from build123d import *

# Parameters (mm, degrees)
BOSS_EXTRUDE1_START       = -0.6
BOSS_EXTRUDE1_DEPTH       = 3.3
BOSS_EXTRUDE1_2_OUTLINE_W = 9.5
BOSS_EXTRUDE1_2_OUTLINE_H = 2.8
BOSS_EXTRUDE1_2_DEPTH     = 0.6
BOSS_EXTRUDE1_3_OUTLINE_R = 0.25
BOSS_EXTRUDE1_3_ANGLE     = 48.590678
SKETCH2_W                 = 12
SKETCH2_H                 = 5
SKETCH2_W_2               = 0.7
SKETCH2_H_2               = 1
BOSS_EXTRUDE2_DEPTH       = 0.4
SKETCH3_W                 = 2.7
SKETCH3_H                 = 9.5
CUT_EXTRUDE1_DEPTH        = 0.6
SKETCH4_W                 = 0.45
SKETCH4_H                 = 1.7
CUT_EXTRUDE2_DEPTH        = 15.612665805
CUT_EXTRUDE3_REACH        = 50.095
SKETCH6_W                 = 0.05
SKETCH6_H                 = 1.7
SKETCH7_W                 = 0.45
SKETCH7_H                 = 1.7
CUT_EXTRUDE4_DEPTH        = 15.612665805
CUT_EXTRUDE5_REACH        = 50.095
SKETCH9_W                 = 0.05
SKETCH9_H                 = 1.7
CUT_EXTRUDE6_REACH        = 50.095
SKETCH11_W                = 0.75
SKETCH11_H                = 0.1
SKETCH12_W                = 0.2
SKETCH12_H                = 1.5
BOSS_EXTRUDE3_DEPTH       = 0.4
CUT_EXTRUDE7_REACH        = 50.095
SKETCH14_W                = 0.75
SKETCH14_H                = 0.1
CUT_EXTRUDE8_REACH        = 50.095
SKETCH16_W                = 0.75
SKETCH16_H                = 0.1
SKETCH17_W                = 0.2
SKETCH17_H                = 1.5
BOSS_EXTRUDE4_DEPTH       = 0.4
CUT_EXTRUDE9_REACH        = 50.095
SKETCH19_W                = 0.75
SKETCH19_H                = 0.1
BOSS_EXTRUDE5_DEPTH       = 9.5
SKETCH21_W                = 0.8
SKETCH21_H                = 0.6
CUT_EXTRUDE10_DEPTH       = 1.8
SKETCH22_W                = 0.8
SKETCH22_H                = 0.6
CUT_EXTRUDE11_DEPTH       = 1.8
SKETCH23_R                = 0.25
BOSS_EXTRUDE6_DEPTH       = 1.35
SKETCH24_R                = 0.25
BOSS_EXTRUDE7_DEPTH       = 1.35
SKETCH25_R                = 0.25
BOSS_EXTRUDE8_DEPTH       = 1.35
SKETCH26_R                = 0.25
BOSS_EXTRUDE9_DEPTH       = 1.35
SKETCH27_R                = 0.25
BOSS_EXTRUDE10_DEPTH      = 1.35
BOSS_EXTRUDE11_DEPTH      = 0.5
BOSS_EXTRUDE12_DEPTH      = 0.5
SKETCH30_R                = 0.25
BOSS_EXTRUDE13_DEPTH      = 1.35
SKETCH31_W                = 0.25
SKETCH31_H                = 2.4
SKETCH32_W                = 0.25
SKETCH32_H                = 2.4
SKETCH33_W                = 0.25
SKETCH33_H                = 2.4
SKETCH34_W                = 0.25
SKETCH34_H                = 2.4
SKETCH35_W                = 0.25
SKETCH35_H                = 2.4
SKETCH36_W                = 0.25
SKETCH36_H                = 2.4


with BuildPart() as part:
    # Boss-Extrude1: read off the stored shape, not the designer's step
    # Boss-Extrude1 outline → Boss-Extrude1 (new body)
    with BuildSketch(Plane(origin=(41.85, 0, 0), x_dir=(0, 0, -1), z_dir=(1, 0, 0)).offset(BOSS_EXTRUDE1_START)):
        Polygon((-4.75, 12.8), (-6, 12.8), (-6, 7.8), (6, 7.8), (6, 12.8), (4.75, 12.8), (4.75, 10), (-4.75, 10), align=None)
    extrude(amount=BOSS_EXTRUDE1_DEPTH)

    # Boss-Extrude1 2 outline → Boss-Extrude1 2 (add)
    with BuildSketch(Plane(origin=(41.85, 0, 0), x_dir=(0, 0, -1), z_dir=(1, 0, 0)).offset(BOSS_EXTRUDE1_START)):
        with Locations((0, 11.4)):
            Rectangle(BOSS_EXTRUDE1_2_OUTLINE_W, BOSS_EXTRUDE1_2_OUTLINE_H)
    extrude(amount=BOSS_EXTRUDE1_2_DEPTH)

    # Boss-Extrude1 3 outline → Boss-Extrude1 3 (revolve)
    with BuildSketch(Plane(origin=(41.95, 7.65, 0), x_dir=(-0.6614338946121362, 0.7500034686974597, 0), z_dir=(0.7500034686974597, 0.6614338946121362, 0))):
        with Locations((0.45, 2.25)):
            Circle(BOSS_EXTRUDE1_3_OUTLINE_R)
        with Locations((0.45, -2.25)):
            Circle(BOSS_EXTRUDE1_3_OUTLINE_R)
        with Locations((0.45, -0.75)):
            Circle(BOSS_EXTRUDE1_3_OUTLINE_R)
        with Locations((0.45, 0.75)):
            Circle(BOSS_EXTRUDE1_3_OUTLINE_R)
        with Locations((0.45, 3.75)):
            Circle(BOSS_EXTRUDE1_3_OUTLINE_R)
        with Locations((0.45, -3.75)):
            Circle(BOSS_EXTRUDE1_3_OUTLINE_R)
    revolve(axis=Axis((41.95, 7.65, 0), (0, 0, 1)), revolution_arc=BOSS_EXTRUDE1_3_ANGLE)

    # Sketch2 → Boss-Extrude2 (add)
    with BuildSketch(Plane(origin=(44.55, 0, 0), x_dir=(0, 0, -1), z_dir=(1, 0, 0))):
        with Locations((0, 10.3)):
            Rectangle(SKETCH2_W, SKETCH2_H)
        with Locations((4.4, 10.5)):
            Rectangle(SKETCH2_W_2, SKETCH2_H_2, mode=Mode.SUBTRACT)
        with Locations((-4.4, 10.5)):
            Rectangle(SKETCH2_W_2, SKETCH2_H_2, mode=Mode.SUBTRACT)
    extrude(amount=BOSS_EXTRUDE2_DEPTH)

    # Sketch3 → Cut-Extrude1 (cut)
    with BuildSketch(Plane(origin=(0, 10, 0), x_dir=(-1, 0, 0), z_dir=(0, 1, 0))):
        with Locations((-43.2, 0)):
            Rectangle(SKETCH3_W, SKETCH3_H)
    extrude(amount=-CUT_EXTRUDE1_DEPTH, mode=Mode.SUBTRACT)

    # Sketch4 → Cut-Extrude2 (cut, through all)
    with BuildSketch(Plane(origin=(44.95, 0, 0), x_dir=(0, 0, -1), z_dir=(1, 0, 0))):
        with Locations((-5.775, 10.85)):
            Rectangle(SKETCH4_W, SKETCH4_H)
    extrude(amount=-CUT_EXTRUDE2_DEPTH, mode=Mode.SUBTRACT)

    # Sketch6 → Cut-Extrude3 (cut, up to next)
    with BuildSketch(Plane(origin=(0, 0, 5.35), x_dir=(-1, 0, 0), z_dir=(0, 0, -1)), mode=Mode.PRIVATE) as cut_extrude3_sk1:
        with Locations((-44.925, 10.85)):
            Rectangle(SKETCH6_W, SKETCH6_H)
    cut_extrude3_tool1 = extrude(cut_extrude3_sk1.sketch, amount=-CUT_EXTRUDE3_REACH, mode=Mode.PRIVATE) & part.part
    add(cut_extrude3_tool1.solids().sort_by_distance((44.925, 10.85, 5.35))[0], mode=Mode.SUBTRACT)

    # Sketch7 → Cut-Extrude4 (cut, through all)
    with BuildSketch(Plane(origin=(44.95, 0, 0), x_dir=(0, 0, -1), z_dir=(1, 0, 0))):
        with Locations((5.775, 10.85)):
            Rectangle(SKETCH7_W, SKETCH7_H)
    extrude(amount=-CUT_EXTRUDE4_DEPTH, mode=Mode.SUBTRACT)

    # Sketch9 → Cut-Extrude5 (cut, up to next)
    with BuildSketch(Plane.XY.offset(-5.35), mode=Mode.PRIVATE) as cut_extrude5_sk1:
        with Locations((44.925, 10.85)):
            Rectangle(SKETCH9_W, SKETCH9_H)
    cut_extrude5_tool1 = extrude(cut_extrude5_sk1.sketch, amount=-CUT_EXTRUDE5_REACH, mode=Mode.PRIVATE) & part.part
    add(cut_extrude5_tool1.solids().sort_by_distance((44.925, 10.85, -5.35))[0], mode=Mode.SUBTRACT)

    # Sketch11 → Cut-Extrude6 (cut, up to next)
    with BuildSketch(Plane.XY.offset(-5.35), mode=Mode.PRIVATE) as cut_extrude6_sk1:
        with Locations((41.625, 10.05)):
            Rectangle(SKETCH11_W, SKETCH11_H)
    cut_extrude6_tool1 = extrude(cut_extrude6_sk1.sketch, amount=-CUT_EXTRUDE6_REACH, mode=Mode.PRIVATE) & part.part
    add(cut_extrude6_tool1.solids().sort_by_distance((41.625, 10.05, -5.35))[0], mode=Mode.SUBTRACT)

    # Sketch12 → Boss-Extrude3 (add)
    with BuildSketch(Plane(origin=(0, 0, -5.55), x_dir=(-1, 0, 0), z_dir=(0, 0, -1))):
        with Locations((-41.35, 10.85)):
            Rectangle(SKETCH12_W, SKETCH12_H)
    extrude(amount=BOSS_EXTRUDE3_DEPTH)

    # Sketch14 → Cut-Extrude7 (cut, up to next)
    with BuildSketch(Plane.XY.offset(-5.35), mode=Mode.PRIVATE) as cut_extrude7_sk1:
        with Locations((41.625, 11.65)):
            Rectangle(SKETCH14_W, SKETCH14_H)
    cut_extrude7_tool1 = extrude(cut_extrude7_sk1.sketch, amount=-CUT_EXTRUDE7_REACH, mode=Mode.PRIVATE) & part.part
    add(cut_extrude7_tool1.solids().sort_by_distance((41.625, 11.65, -5.35))[0], mode=Mode.SUBTRACT)

    # Sketch16 → Cut-Extrude8 (cut, up to next)
    with BuildSketch(Plane(origin=(0, 0, 5.35), x_dir=(-1, 0, 0), z_dir=(0, 0, -1)), mode=Mode.PRIVATE) as cut_extrude8_sk1:
        with Locations((-41.625, 11.65)):
            Rectangle(SKETCH16_W, SKETCH16_H)
    cut_extrude8_tool1 = extrude(cut_extrude8_sk1.sketch, amount=-CUT_EXTRUDE8_REACH, mode=Mode.PRIVATE) & part.part
    add(cut_extrude8_tool1.solids().sort_by_distance((41.625, 11.65, 5.35))[0], mode=Mode.SUBTRACT)

    # Sketch17 → Boss-Extrude4 (add)
    with BuildSketch(Plane.XY.offset(5.55)):
        with Locations((41.35, 10.85)):
            Rectangle(SKETCH17_W, SKETCH17_H)
    extrude(amount=BOSS_EXTRUDE4_DEPTH)

    # Sketch19 → Cut-Extrude9 (cut, up to next)
    with BuildSketch(Plane(origin=(0, 0, 5.35), x_dir=(-1, 0, 0), z_dir=(0, 0, -1)), mode=Mode.PRIVATE) as cut_extrude9_sk1:
        with Locations((-41.625, 10.05)):
            Rectangle(SKETCH19_W, SKETCH19_H)
    cut_extrude9_tool1 = extrude(cut_extrude9_sk1.sketch, amount=-CUT_EXTRUDE9_REACH, mode=Mode.PRIVATE) & part.part
    add(cut_extrude9_tool1.solids().sort_by_distance((41.625, 10.05, 5.35))[0], mode=Mode.SUBTRACT)

    # Sketch20 → Boss-Extrude5 (add)
    with BuildSketch(Plane(origin=(0, 0, 4.75), x_dir=(-1, 0, 0), z_dir=(0, 0, -1))):
        Polygon((-42.9, 9.4), (-44.55, 9.4), (-44.55, 9.7), (-43.2, 9.7), align=None)
    extrude(amount=BOSS_EXTRUDE5_DEPTH)

    # Sketch21 → Cut-Extrude10 (cut)
    with BuildSketch(Plane(origin=(0, 12.8, 0), x_dir=(-1, 0, 0), z_dir=(0, 1, 0))):
        with Locations((-43.65, -5.05)):
            Rectangle(SKETCH21_W, SKETCH21_H)
    extrude(amount=-CUT_EXTRUDE10_DEPTH, mode=Mode.SUBTRACT)

    # Sketch22 → Cut-Extrude11 (cut)
    with BuildSketch(Plane(origin=(0, 12.8, 0), x_dir=(-1, 0, 0), z_dir=(0, 1, 0))):
        with Locations((-43.65, 5.05)):
            Rectangle(SKETCH22_W, SKETCH22_H)
    extrude(amount=-CUT_EXTRUDE11_DEPTH, mode=Mode.SUBTRACT)

    # Sketch23 → Boss-Extrude6 (add)
    with BuildSketch(Plane.XZ.offset(-7.65)):
        with Locations(Location((41.5, 2.25, 0), (0, 0, 90))):
            Circle(SKETCH23_R)
    extrude(amount=BOSS_EXTRUDE6_DEPTH)

    # Sketch24 → Boss-Extrude7 (add)
    with BuildSketch(Plane.XZ.offset(-7.65)):
        with Locations(Location((41.5, -0.75, 0), (0, 0, 90))):
            Circle(SKETCH24_R)
    extrude(amount=BOSS_EXTRUDE7_DEPTH)

    # Sketch25 → Boss-Extrude8 (add)
    with BuildSketch(Plane.XZ.offset(-7.65)):
        with Locations(Location((41.5, -3.75, 0), (0, 0, 90))):
            Circle(SKETCH25_R)
    extrude(amount=BOSS_EXTRUDE8_DEPTH)

    # Sketch26 → Boss-Extrude9 (add)
    with BuildSketch(Plane.XZ.offset(-7.65)):
        with Locations(Location((41.5, -2.25, 0), (0, 0, 90))):
            Circle(SKETCH26_R)
    extrude(amount=BOSS_EXTRUDE9_DEPTH)

    # Sketch27 → Boss-Extrude10 (add)
    with BuildSketch(Plane.XZ.offset(-7.65)):
        with Locations(Location((41.5, 0.75, 0), (0, 0, 90))):
            Circle(SKETCH27_R)
    extrude(amount=BOSS_EXTRUDE10_DEPTH)

    # Sketch28 → Boss-Extrude11 (add)
    with BuildSketch(Plane.XY.offset(6)):
        Polygon((43.35, 7.8), (41.25, 7.8), (41.25, 6.8), (42.75, 6.8), align=None)
    extrude(amount=-BOSS_EXTRUDE11_DEPTH)

    # Sketch29 → Boss-Extrude12 (add)
    with BuildSketch(Plane(origin=(0, 0, -6), x_dir=(-1, 0, 0), z_dir=(0, 0, -1))):
        Polygon((-41.25, 6.8), (-41.25, 7.8), (-43.35, 7.8), (-42.75, 6.8), align=None)
    extrude(amount=-BOSS_EXTRUDE12_DEPTH)

    # Sketch30 → Boss-Extrude13 (add)
    with BuildSketch(Plane.XZ.offset(-7.65)):
        with Locations(Location((41.5, 3.75, 0), (0, 0, 90))):
            Circle(SKETCH30_R)
    extrude(amount=BOSS_EXTRUDE13_DEPTH)

    # Sketch31 → Revolve1 (revolve)
    with BuildSketch(Plane.XY.offset(3.75)):
        with Locations((43.775, 10.9)):
            Rectangle(SKETCH31_W, SKETCH31_H)
    revolve(axis=Axis((43.65, 12.1, 3.75), (0, -1, 0)))

    # Sketch32 → Revolve2 (revolve)
    with BuildSketch(Plane.XY.offset(0.75)):
        with Locations((43.775, 10.9)):
            Rectangle(SKETCH32_W, SKETCH32_H)
    revolve(axis=Axis((43.65, 12.1, 0.75), (0, -1, 0)))

    # Sketch33 → Revolve3 (revolve)
    with BuildSketch(Plane.XY.offset(-2.25)):
        with Locations((43.775, 10.9)):
            Rectangle(SKETCH33_W, SKETCH33_H)
    revolve(axis=Axis((43.65, 12.1, -2.25), (0, -1, 0)))

    # Sketch34 → Revolve4 (revolve)
    with BuildSketch(Plane.XY.offset(-3.75)):
        with Locations((43.775, 10.9)):
            Rectangle(SKETCH34_W, SKETCH34_H)
    revolve(axis=Axis((43.65, 12.1, -3.75), (0, -1, 0)))

    # Sketch35 → Revolve5 (revolve)
    with BuildSketch(Plane.XY.offset(-0.75)):
        with Locations((43.775, 10.9)):
            Rectangle(SKETCH35_W, SKETCH35_H)
    revolve(axis=Axis((43.65, 12.1, -0.75), (0, -1, 0)))

    # Sketch36 → Revolve6 (revolve)
    with BuildSketch(Plane.XY.offset(2.25)):
        with Locations((43.775, 10.9)):
            Rectangle(SKETCH36_W, SKETCH36_H)
    revolve(axis=Axis((43.65, 12.1, 2.25), (0, -1, 0)))


solid = part.part
Source: CAD feature listing. Evaluate the final solid. Frame: model axes, mm. A direction names the side the tool comes from. Round coordinates to 2 decimals unless told otherwise and drop trailing zeros. Write each loop counter-clockwise with the first axis right and the second up, starting at its lowest first coordinate (ties: lowest second). Pieces come first, ordered by that corner, then holes. Notation, with made-up numbers: M 25.25,21.5 L 34.25,21.5 A17 ccw 34.25,54.5 Z; hole C -39,-28.5 d5. An arc over 180 degrees is marked long. One line per item, written item: value. Start each with the question number.
Item 1: Set-up query: faces 1 (the flat face through (43, 11, -5.55)), 2 (the flat face through (43, 11, 5.55)), 3 (the flat face through (42, 7, -5.5)), 4 (the flat face through (44, 9.7, 0)). Return all of +Z, -Z, +X, -X, +Y, -Y with unobstructed straight access to the full face (end or side cutting, diameter ignored); none if empty.
Item 2: Mould query, pull axis Z, two halves, no side actions, for faces 5 (the flat face through (41.25, 10, 0)), 6 (the flat face through (43, 9, 6)), 7 (the flat face through (43, 11, 4.75)). Classes: pulls with the +Z half, pulls with the -Z half, needs draft (parallel to the pull), parting line crosses it, or undercut.
Item 3: Ray query, L1, parallel to Z at x = 42.7, y = 7.25; L2, parallel to Z at x = 42.35, y = 12; L3, parallel to X at y = 10.75, z = -3. Return the intervals inside material, ascending. Write a range as from..to.
Item 4: Section query A-A (z = -4.25). Return the cut outline in (x, y), plus the area to 3 significant figures.
Item 5: Section query D-D (z = 1.75). Return the cut outline in (x, y), plus the area to 3 significant figures.
Item 6: Section query B-B (y = 10.75). Return the cut outline in (x, z).
Item 7: Pin query (flat end, axial travel): pin 1 (0.9 mm diameter, centred on x = 43, y = 11, fed in from +Z). Return the tip coordinate at first contact, or that it passes through.
Result set:
1. face 1: -Z, +X
1. face 2: +Z, +X
1. face 3: +X, -X, -Y
1. face 4: +Y
2. face 5: needs draft
2. face 6: pulls with the +Z half
2. face 7: undercut
3. L1: z = -6..-5.5, 5.5..6
3. L2: z = -6..-4.75, 4.75..6
3. L3: x = 41.25..41.85, 44.55..44.95
4. outline: M 41.25,7.8 L 44.95,7.8 L 44.95,10 L 44.55,10 L 44.55,9.7 L 43.2,9.7 L 42.9,9.4 L 41.85,9.4 L 41.85,12.8 L 41.25,12.8 Z; M 44.55,11 L 44.95,11 L 44.95,12.8 L 44.55,12.8 Z
4. area: 9.37 mm²
5. outline: M 41.25,7.8 L 44.95,7.8 L 44.95,12.8 L 44.55,12.8 L 44.55,9.7 L 43.2,9.7 L 42.9,9.4 L 41.85,9.4 L 41.85,12.8 L 41.25,12.8 Z
5. area: 9.77 mm²
6. outline: M 41.25,-5.95 L 41.45,-5.95 L 41.45,-5.55 L 44.9,-5.55 L 44.9,-5.35 L 44.95,-5.35 L 44.95,-4.75 L 41.85,-4.75 L 41.85,4.75 L 44.95,4.75 L 44.95,5.35 L 44.9,5.35 L 44.9,5.55 L 41.45,5.55 L 41.45,5.95 L 41.25,5.95 Z; C 43.65,-3.75 d0.5; C 43.65,-2.25 d0.5; C 43.65,-0.75 d0.5; C 43.65,0.75 d0.5; C 43.65,2.25 d0.5; C 43.65,3.75 d0.5; M 44.55,-4.05 L 44.95,-4.05 L 44.95,4.05 L 44.55,4.05 Z
7. pin 1: stops at z = 5.55
